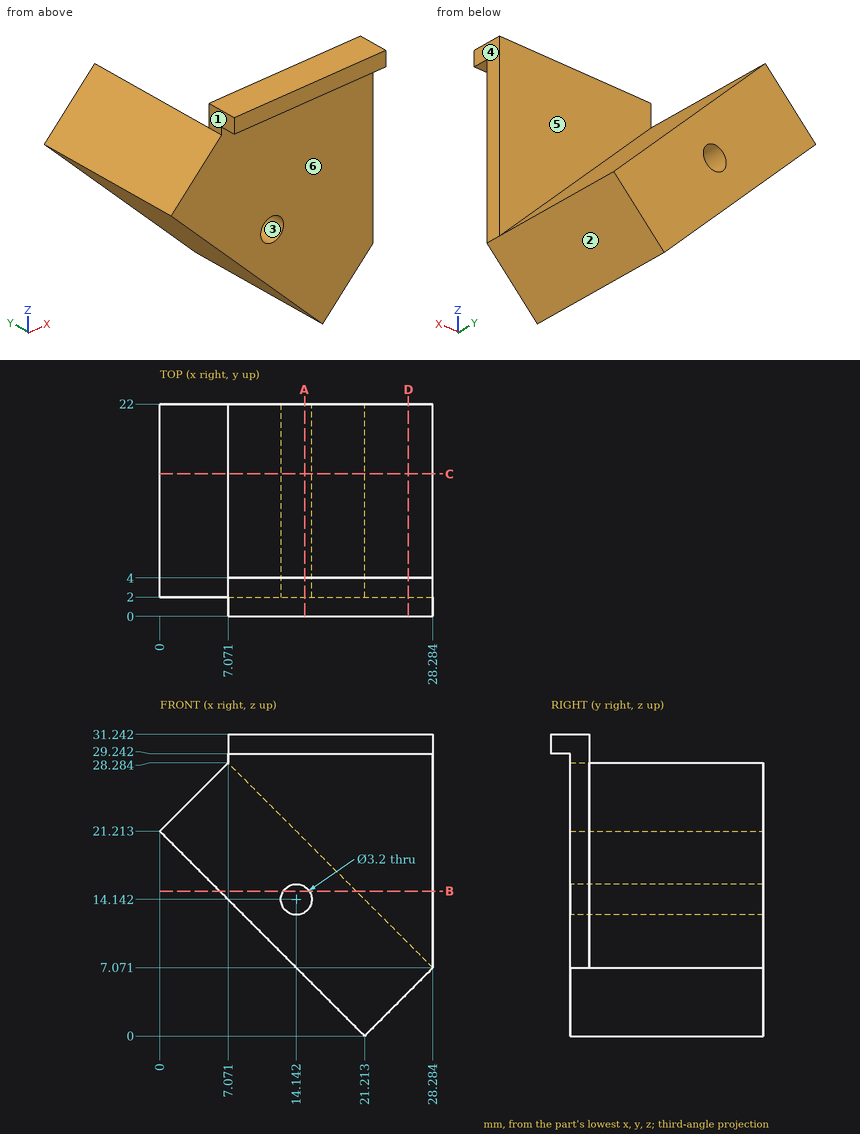
The figure shows three views and two pictorial views of one solid part (mm, origin at its lowest corner). Answer the questions. A direction names the side the tool comes from. Coordinates: 2 decimals unless noted, no trailing zeros. Write each loop counter-clockwise with the first axis right and the second up, starting at its lowest first coordinate (ties: lowest second). Pieces come first, ordered by that corner, then holes.
1. Flat-ended cylindrical pins translate along their axes: pin 1 (5 mm diameter, centred on x = 14, z = 27, fed in from +Y); pin 2 (12 mm diameter, centred on x = 6.5, z = 15, fed in from -Y); pin 3 (1.5 mm diameter, centred on x = 4.5, y = 7.5, fed in from -Z); pin 4 (1.9 mm diameter, centred on x = 14.14, z = 14.14, fed in from -Y). Find the tip coordinate at first contact, or state that the pin passes through.
Results list:
pin 1: stops at y = 4
pin 2: stops at y = 2
pin 3: stops at z = 15.96
pin 4: passes through
2. For the marked faces 4, 5 and 6, determine the directions among +Z, -Z, +X, -X, +Y, -Y from which every point of the face is accessible in a straight line to the end or side of a thin tool.
Results list:
face 4: +Z, -Z, +X, +Y, -Y
face 5: +Z, +X, +Y
face 6: -Z, +X, -X, -Y
3. Consider line 1 along Y through (x, z) = (7, 27); line 2 along Y through (x, z) = (23.5, 18); line 3 along Z through (x, y) = (13.75, 11) (1 decimal). Determine where each line is inside the solid, lowest interval first.
Results list:
line 1: y = 2 to 22
line 2: y = 2 to 4
line 3: z = 7.5 to 12.6, 15.7 to 21.6
4. The part is cut by section D-D, the plane x = 25.75. Write down the section's boundary in (y, z) (1 decimal).
Results list:
outline: (0, 29.2) - (2, 29.2) - (2, 4.5) - (22, 4.5) - (22, 9.6) - (4, 9.6) - (4, 31.2) - (0, 31.2) - close
5. For a pull along X with two mould halves and no side action, classify the marked faces 1, 2 and 3 as +X half, -X half, draft (parallel to the pull), parting line (faces both ways), or undercut.
Results list:
face 1: -X half
face 2: +X half
face 3: undercut
6. The part is cut by section B-B, the plane z = 15. Write down the section's boundary in (x, y) (1 decimal), and give its area (3 significant figures).
Results list:
outline: (6.2, 2) - (12.8, 2) - (12.8, 22) - (6.2, 22) - close; (15.5, 2) - (28.3, 2) - (28.3, 4) - (20.4, 4) - (20.4, 22) - (15.5, 22) - close
area: 245 mm2
7. The part is cut by section A-A, the plane x = 15. Write down the section's boundary in (y, z) (1 decimal).
Results list:
outline: (0, 29.2) - (2, 29.2) - (2, 15.5) - (22, 15.5) - (22, 20.4) - (4, 20.4) - (4, 31.2) - (0, 31.2) - close; (2, 6.2) - (22, 6.2) - (22, 12.8) - (2, 12.8) - close
8. The part is cut by section C-C, the plane y = 14.75. Write down the section's boundary in (x, z), and give its area (3 significant figures).
Results list:
outline: (0, 21.21) - (21.21, 0) - (28.28, 7.07) - (7.07, 28.28) - close; hole circle Ø3.2 at (14.14, 14.14)
area: 292 mm2
